Study the drawing (mm; zero at the part's minimum x, y, z) and answer. A direction names the side the tool comes from. Give positions to 0.01 mm unless a question says otherwise; leave off trailing zeros. Loops run counter-clockwise (first coordinate to the right, second up) from the corner with the lowest first, then second, coordinate; pieces in that order, holes last. Notation, with made-up numbers: (-40, 46) - (8, 46) arc R14 cw to (8, 62) - close; hole circle Ø5 at (-32, 60). An arc over 180 degrees is marked (long way). Write item = value, one per line. Start each with the question number.
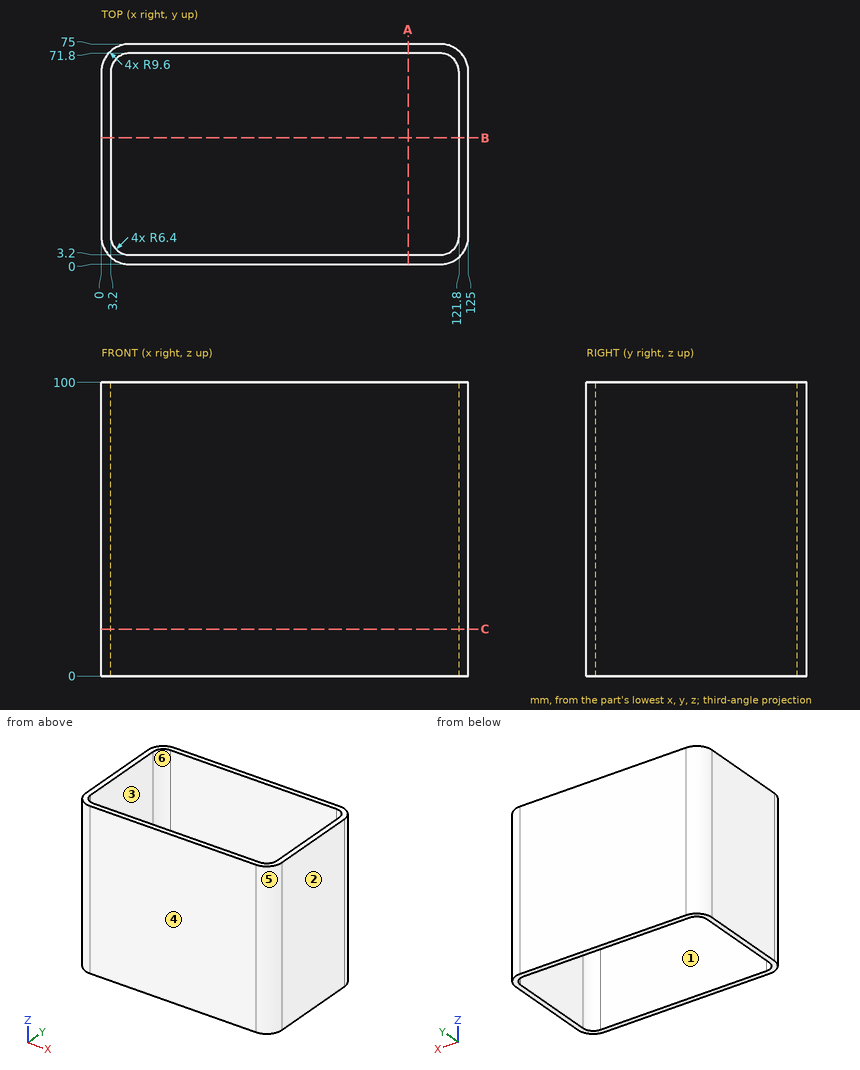
1. A tool of negligible diameter and unlimited length cuts with its end or side. For the marked faces 5 and 6, from which of +Z, -Z, +X, -X, +Y, -Y can it reach the whole face along a straight path? Write none if from no direction.
2. Consider line 1 along Y through (x, z) = (112, 18.5); line 2 along X through (y, z) = (48.5, 18); line 3 along Y through (x, z) = (117.5, 10.5). Determine where each line is inside the solid, lowest interval first. Write a range as [from, to].
3. A cutting plane is placed at C-C on z = 16. Give the vertices of the cut face in (x, y).
4. A cutting plane is placed at A-A on x = 104.5. Give the vertices of the cut face in (y, z), and give its area (3 significant figures).
5. For a pull along Y with two mould halves and no side action, classify the marked faces 1, 2, 3 and 4 as released by +Y, released by -Y, zero draft, split by the parting line, or undercut.
6. A cutting plane is placed at B-B on y = 43. Give the vertices of the cut face in (x, z), and give its area (3 significant figures).
Reply:
q1.face_5 = +Z, -Z, +X, -Y
q1.face_6 = +Z, -Z
q2.line_1 = [0, 3.2], [71.8, 75]
q2.line_2 = [0, 3.2], [121.8, 125]
q2.line_3 = [0.23, 3.55], [71.45, 74.77]
q3.outline = (0, 9.6) arc R9.6 ccw to (9.6, 0) - (115.4, 0) arc R9.6 ccw to (125, 9.6) - (125, 65.4) arc R9.6 ccw to (115.4, 75) - (9.6, 75) arc R9.6 ccw to (0, 65.4) - close; hole (3.2, 9.6) arc R6.4 ccw to (9.6, 3.2) - (115.4, 3.2) arc R6.4 ccw to (121.8, 9.6) - (121.8, 65.4) arc R6.4 ccw to (115.4, 71.8) - (9.6, 71.8) arc R6.4 ccw to (3.2, 65.4) - close
q4.outline = (0, 0) - (3.2, 0) - (3.2, 100) - (0, 100) - close; (71.8, 0) - (75, 0) - (75, 100) - (71.8, 100) - close
q4.area = 640 mm^2
q5.face_1 = undercut
q5.face_2 = zero draft
q5.face_3 = undercut
q5.face_4 = released by -Y
q6.outline = (0, 0) - (3.2, 0) - (3.2, 100) - (0, 100) - close; (121.8, 0) - (125, 0) - (125, 100) - (121.8, 100) - close
q6.area = 640 mm^2
